The model under review builds one solid part; all positions refer to its coordinate system, in mm. Round coordinates to 2 decimals unless told otherwise and drop trailing zeros. Order: outer loops, then holes, each group sorted by start corner. A loop starts at its lowest first (then second) coordinate and runs counter-clockwise, first axis right, second up.
1) Clearance check with flat-ended pins moving along their axes: P1, Ø2, axis at x = 5, z = 1.5, coming from the +Y side; P2, Ø5, axis at y = 30, z = -16, coming from the -X side; P3, Ø24, axis at x = 0, z = 0, coming from the +Y side; P4, Ø6, axis at x = -4.5, y = -4, coming from the +Z side. State where each tip first meets the part, or that it passes through.
2) Consider section C-C (y = -21). Give the boundary of the cut face in (x, z), then the cut area to 3 significant figures.
3) Mouldability with a two-part tool opening along X and no side actions: class faces 1 (the face through (0.33, 0.98, -7.493)), 2 (the face through (8.86, 0.84, 28.14)), 3 (the face through (0, 70, 8)) as pulls with the +X half, pulls with the -X half, needs draft (parallel to the pull), parting line crosses it, or undercut.
4) Consider section A-A (z = 0). Give the boundary of the cut face in (x, y).
5) Consider section B-B (x = 0). Give the boundary of the cut face in (y, z).
6) To check wall thickness, follow L1, parallel to X at y = -3, z = 0; L2, parallel to Z at x = 2.5, y = 7; L3, parallel to Z at x = 4, y = 26. State the ranges of each line that lie inside material, in increasing order.
from build123d import *

# Parameters (mm, degrees)
SKETCH1_R           = 29.5
BOSS_EXTRUDE1_DEPTH = 70
FILLET1_R           = 10
SKETCH2_R           = 7.5
CUT_EXTRUDE1_DEPTH  = 147.083880034


with BuildPart() as part:
    # Sketch1 → Boss-Extrude1 (new, symmetric)
    with BuildSketch(Plane(origin=(0, 0, 0), x_dir=(1, 0, 0), z_dir=(0, 1, 0))):
        with Locations(Location((0, 0, 0), (0, 0, 270))):
            Circle(SKETCH1_R)
    extrude(amount=BOSS_EXTRUDE1_DEPTH, both=True)

    # Fillet1
    fillet1_edges = [part.edges().sort_by_distance(p)[0] for p in [
        (0, -70, -29.5),
        (0, 70, -29.5),
    ]]
    fillet(fillet1_edges, radius=FILLET1_R)

    # Sketch2 → Cut-Extrude1 (cut, through all)
    with BuildSketch(Plane(origin=(0, 70, 0), x_dir=(1, 0, 0), z_dir=(0, 1, 0))):
        with Locations(Location((0, 0, 0), (0, 0, 270))):
            Circle(SKETCH2_R)
    extrude(amount=-CUT_EXTRUDE1_DEPTH, mode=Mode.SUBTRACT)


solid = part.part
Answer below:
1. P1: passes through
1. P2: stops at x = -26.23
1. P3: stops at y = 70
1. P4: stops at z = 29.46
2. outline: circle Ø59 at (0, 0); hole circle Ø15 at (0, 0)
2. area: 2,560 mm2
3. face 1: undercut
3. face 2: parting line crosses it
3. face 3: needs draft
4. outline: (-29.5, -60) arc R10 ccw to (-19.5, -70) - (-7.5, -70) - (-7.5, 70) - (-19.5, 70) arc R10 ccw to (-29.5, 60) - close; (7.5, -70) - (19.5, -70) arc R10 ccw to (29.5, -60) - (29.5, 60) arc R10 ccw to (19.5, 70) - (7.5, 70) - close
5. outline: (-70, -19.5) arc R10 ccw to (-60, -29.5) - (60, -29.5) arc R10 ccw to (70, -19.5) - (70, -7.5) - (-70, -7.5) - close; (-70, 7.5) - (70, 7.5) - (70, 19.5) arc R10 ccw to (60, 29.5) - (-60, 29.5) arc R10 ccw to (-70, 19.5) - close
6. L1: x = -29.5 to -7.5, 7.5 to 29.5
6. L2: z = -29.39 to -7.07, 7.07 to 29.39
6. L3: z = -29.23 to -6.34, 6.34 to 29.23
